Read the model definition and answer for the solid it produces. Units are mm, in the model's axes. Face numbers are marked on the shaded views. Coordinates: 2 decimals unless noted, no trailing zeros. Write each loop counter-clockwise with the first axis right and the second up, starting at its lowest first coordinate (ties: lowest second). Pieces come first, ordered by that corner, then holes. Notation, with made-up numbers: (14.5, 72.5) -> (30.5, 72.5) arc R22 cw to (30.5, 79.5) -> close; hole circle Ø6 at (-7, 77.25). An arc over 180 degrees is marked (long way). Answer in a Markdown table with one row per item. Add a question column.
Item 1: Given pin 1 Ø3 at (x, y) = (4, 8) entering from -Z; pin 2 Ø1.5 at (x, z) = (5, -3.5) entering from -Y; pin 3 Ø5 at (x, y) = (16, -6.5) entering from -Z, each flat-ended and moving along its own axis, determine where each tip first touches the part or whether it passes through.
Item 2: Section D-D on z = -9 is taken. Write down the section's boundary in (x, y), then the cut area to 3 significant figures.
Item 3: Section A-A on y = 1.75 is taken. Write down the section's boundary in (x, z).
Item 4: Section B-B on z = 0 is taken. Write down the section's boundary in (x, y).
Item 5: Straight lines are drawn through the part: line 1 (Y direction, x = 16, z = 0); line 2 (Z direction, x = 14.75, y = -0.25); line 3 (Z direction, x = 16.5, y = -12). For each, find the intervals that lie inside material, in ascending order. Write a range as from..to.
Item 6: For a pull along Y with two mould halves and no side action, classify the marked faces 1, 2 and 3 as +Y half, -Y half, draft (parallel to the pull), parting line (faces both ways), or undercut.
Item 7: Section C-C on z = 7.75 is taken. Write down the section's boundary in (x, y).
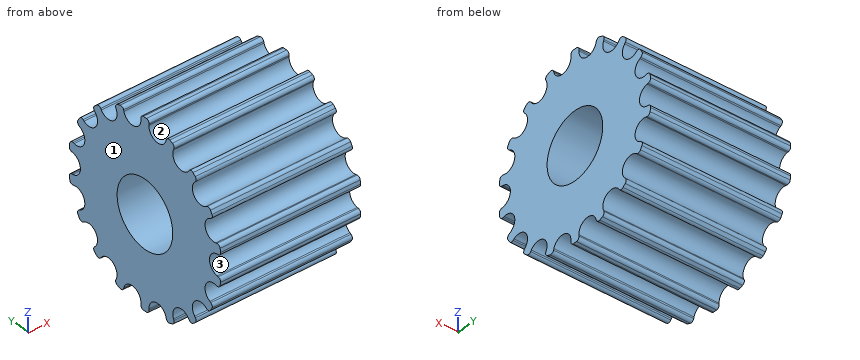
```python
from build123d import *

# Parameters (mm, degrees)
CHAMFER_1_SIZE           = 1
SKETCH_4_W               = 2
SKETCH_4_H               = 1
CUT_EXTRUDE_1_DEPTH      = 35.092374778
CUT_EXTRUDE_2_REACH      = 36.092
PATTERN_CIRCULAR_3_COUNT = 18
SKETCH_7_R               = 16.570868864
CUT_EXTRUDE_3_DEPTH      = 7
SKETCH_8_R               = 8.79239993
EXTRUDE_1_DEPTH          = 21
SKETCH_9_R               = 5
CUT_EXTRUDE_4_DEPTH      = 21


with BuildPart() as part:
    # 草图1 → 旋转1 (revolve)
    with BuildSketch(Plane.XY, mode=Mode.PRIVATE) as revolve_1_sk:
        Polygon((0, 2.7506), (0, 13.753), (28, 13.753), (28, 5.5012), (20, 5.5012), (20, 2.7506), align=None)
    revolve(revolve_1_sk.sketch.rotate(Axis((0, 0, 0), (1, 0, 0)), 90), axis=Axis((0, 0, 0), (1, 0, 0)))

    # 倒角1
    chamfer_1_edges = [part.edges().sort_by_distance(p)[0] for p in [
        (20, 0, -2.7506),
        (0, 0, -2.7506),
    ]]
    chamfer(chamfer_1_edges, length=CHAMFER_1_SIZE)

    # 草图4 → 切除-拉伸1 (cut, through all)
    with BuildSketch(Plane.ZY):
        with Locations((0, 3.062381775)):
            Rectangle(SKETCH_4_W, SKETCH_4_H)
    extrude(amount=-CUT_EXTRUDE_1_DEPTH, mode=Mode.SUBTRACT)

    # 草图6 → 切除-拉伸2 (cut, up to next)
    with BuildSketch(Plane(origin=(0, 0, 0), x_dir=(0, 0, -1), z_dir=(1, 0, 0)), mode=Mode.PRIVATE) as cut_extrude_2_sk1:
        with BuildLine():
            Line((1.574067282, 13.17215513), (1.548371997, 12.962883824))
            ThreePointArc((1.548371997, 12.962883824), (0, 11.593), (-1.548371997, 12.962883824))
            Line((-1.548371997, 12.962883824), (-1.574067282, 13.17215513))
            ThreePointArc((-1.574067282, 13.17215513), (-1.761240253, 13.496717776), (-2.124642597, 13.587895453))
            ThreePointArc((-2.124642597, 13.587895453), (-2.36143787, 13.548749765), (-2.597513963, 13.505477785))
            Line((-2.597513963, 13.505477785), (-2.794161951, 15.107047128))
            ThreePointArc((-2.794161951, 15.107047128), (0, 15.363274844), (2.794161951, 15.107047128))
            Line((2.794161951, 15.107047128), (2.597513963, 13.505477785))
            ThreePointArc((2.597513963, 13.505477785), (2.36143787, 13.548749765), (2.124642597, 13.587895453))
            ThreePointArc((2.124642597, 13.587895453), (1.761240253, 13.496717776), (1.574067282, 13.17215513))
        make_face()
    cut_extrude_2_tool1 = extrude(cut_extrude_2_sk1.sketch, amount=CUT_EXTRUDE_2_REACH, mode=Mode.PRIVATE) & part.part
    cut_extrude_2 = cut_extrude_2_tool1.solids().sort_by_distance((0, 13.819423, 0))[0]
    add(cut_extrude_2, mode=Mode.SUBTRACT)

    # 阵列(圆周)3: 切除-拉伸2 ×18 about axis
    pattern_circular_3_axis = Axis((0, 0, 0), (1, 0, 0))
    for i in range(1, PATTERN_CIRCULAR_3_COUNT):
        add(cut_extrude_2.rotate(pattern_circular_3_axis, i * 360 / PATTERN_CIRCULAR_3_COUNT), mode=Mode.SUBTRACT)

    # 草图7 → 切除-拉伸3 (cut)
    with BuildSketch(Plane(origin=(28, 0, 0), x_dir=(0, 0, -1), z_dir=(1, 0, 0))):
        Circle(SKETCH_7_R)
    extrude(amount=-CUT_EXTRUDE_3_DEPTH, mode=Mode.SUBTRACT)

    # 草图8 → 凸台-拉伸1 (add)
    with BuildSketch(Plane(origin=(21, 0, 0), x_dir=(0, 0, -1), z_dir=(1, 0, 0))):
        Circle(SKETCH_8_R)
    extrude(amount=-EXTRUDE_1_DEPTH)

    # 草图9 → 切除-拉伸4 (cut)
    with BuildSketch(Plane(origin=(21, 0, 0), x_dir=(0, 0, -1), z_dir=(1, 0, 0))):
        Circle(SKETCH_9_R)
    extrude(amount=-CUT_EXTRUDE_4_DEPTH, mode=Mode.SUBTRACT)


solid = part.part
```
Results below:
| question | item | result |
|---|---|---|
| 1 | pin 1 | stops at z = -10.81 |
| 1 | pin 2 | stops at y = -13.46 |
| 1 | pin 3 | stops at z = -13.04 |
| 2 | outline | (0, -8.61) -> (21, -8.61) -> (21, 8.61) -> (0, 8.61) -> close |
| 2 | area | 362 mm2 |
| 3 | outline | (0, -11.49) -> (21, -11.49) -> (21, -4.68) -> (0, -4.68) -> close; (0, 4.68) -> (21, 4.68) -> (21, 11.49) -> (0, 11.49) -> close |
| 4 | outline | (0, -11.59) -> (21, -11.59) -> (21, -5) -> (0, -5) -> close; (0, 5) -> (21, 5) -> (21, 11.59) -> (0, 11.59) -> close |
| 5 | line 1 | y = -11.59..-5, 5..11.59 |
| 5 | line 2 | z = -13.75..-4.99, 4.99..13.75 |
| 5 | line 3 | z = -6.72..-6.12, -2.98..-1.05, 1.05..2.98, 6.12..6.72 |
| 6 | face 1 | draft |
| 6 | face 2 | undercut |
| 6 | face 3 | -Y half |
| 7 | outline | (0, -8.68) -> (21, -8.68) -> (21, 8.68) -> (0, 8.68) -> close |
